Input: part model. Units: mm. Frame: model coordinates. A direction names the side the tool comes from. Coordinates: 2 decimals unless noted, no trailing zeros. Loops run counter-clockwise (first coordinate to the right, second up) from the corner with the lowest first, then second, coordinate; pieces in that order, holes last. Notation, with made-up numbers: (32.5, 85.25) - (76.5, 85.25) arc R26 cw to (76.5, 120.25) - close; hole circle Ø3 at (-9, 63). An arc over 180 degrees is marked (long way). Use a Markdown table: item, result. Add a question column.
1. Section query C-C on y = 4. Return the cut outline in (x, z) (3 decimals).
2. Section query A-A on x = -50.8. Return the cut outline in (y, z), then the cut area to 3 significant figures.
3. Section query B-B on z = -15.24. Return the cut outline in (x, y), then the cut area to 3 significant figures.
4. Ray query, L1, parallel to Z at x = -35.56, y = 1; L2, parallel to X at y = 8.5, z = -30.5; L3, parallel to X at y = 9.75, z = -4. Return the intervals inside material, ascending. Write a range as [from, to].
5. Contact query for flat-ended pins moving along their axis: P1, Ø2.5, axis at y = 6.5, z = 2.5, coming from the -X side; P2, Ø0.6, axis at x = -3.5, z = -4.5, coming from the +Y side; P3, Ø2.5, axis at y = 6, z = -54.5, coming from the +X side. Output: stop coordinate, or through.
6. Draft query along Y for faces 5 (the face through (-3.5, 6, -3)), 6 (the face through (-34.93, 10.09, 1.08)), 7 (the face through (-51, 10, -42)). Return one class per face: released by +Y, released by -Y, zero draft, split by the parting line, or undercut.
7. Access query for faces 1 (the face through (-8, 8, 2)), 2 (the face through (-44.34, 7, -2)), 3 (the face through (-42.565, 6, 1)), 4 (the face through (-38, 7, -10)). Directions: +Z, -Z, +X, -X, +Y, -Y. A direction counts if a zero-diameter tool reaches every point of the face in a straight line with its end or side. Return the directions, or none.
8. Section query D-D on z = -49.5. Return the cut outline in (x, y).
Autodesk Inventor part; units mm, degrees
ref_plane "YZ Plane" through (0, 0, 0) normal (1, 0, 0) x (0, 1, 0)
ref_plane "XZ Plane" through (0, 0, 0) normal (0, 1, 0) x (-1, 0, 0)
ref_plane "XY Plane" through (0, 0, 0) normal (0, 0, 1) x (1, 0, 0)
sketch "Sketch1" plane through (0, 0, 0) normal (0, 1, 0) x (-1, 0, 0)
  line L0 (0, 0) -> (53.34, 0)
  line L1 (53.34, 0) -> (53.34, -66.04)
  line L2 (0, -66.04) -> (0, 0)
  circle A0 centre (50.8, -15.24) radius 1.6
  circle A1 centre (2.54, -15.24) radius 1.6
  circle A2 centre (35.56, -66.04) radius 1.6
  circle A3 centre (7.62, -66.04) radius 1.6
  line L3 (2.54, -66.04) -> (5.08, -68.58)
  line L4 (5.08, -68.58) -> (38.02, -68.58)
  line L5 (38.02, -68.58) -> (40.56, -66.04)
  line L6 (53.34, -66.04) -> (40.56, -66.04)
  line L7 (2.54, -66.04) -> (0, -66.04)
  dimension "d0" = 66.04
  dimension "d1" = 53.34
  dimension "d2" = 3.2
  dimension "d3" = 2.54
  dimension "d4" = 2.54
  dimension "d5" = 45.72
  dimension "d6" = 17.78
  dimension "d7" = 2.54
  dimension "d8" = 2.54
  dimension "d9" = 2.54
  dimension "d10" = 2.54
  dimension "d11" = 15.24
  dimension "d12" = 15.24
  dimension "d13" = 5
extrude "Extrusion1" add sketch "Sketch1" along normal blind 1.5
sketch "Sketch2" plane through (0, 1.5, 0) normal (0, 1, 0) x (1, 0, 0)
  line L0 (-44.34, 10) -> (-32.34, 10)
  line L1 (-32.34, 10) -> (-32.34, -6.5)
  line L2 (-32.34, -6.5) -> (-44.34, -6.5)
  line L3 (-44.34, -6.5) -> (-44.34, 10)
  line L4 (-53.34, 0) -> (0, 0)
  line L5 (-53.34, 66.04) -> (-53.34, 0)
  dimension "d16" = 12
  dimension "d17" = 16.5
  dimension "d18" = 6.5
  dimension "d41" = 9
extrude "Extrusion2" add sketch "Sketch2" along normal blind 11
sketch "Sketch3" plane through (-44.34, 1.5, 6.5) normal (0, 0, 1) x (1, 0, 0)
  line L0 (3.25, 7.025) -> (8.75, 7.025)
  line L1 (8.75, 7.025) -> (8.75, 3.975)
  line L2 (8.75, 3.975) -> (3.25, 3.975)
  line L3 (3.25, 3.975) -> (3.25, 7.025)
  line L4 (1.775, 1.61) -> (10.225, 1.61)
  line L5 (10.225, 1.61) -> (10.225, 7.775)
  line L6 (8.61, 9.39) -> (3.39, 9.39)
  line L7 (1.775, 7.775) -> (1.775, 1.61)
  line L8 (1.775, 7.775) -> (3.39, 9.39)
  line L9 (8.61, 9.39) -> (10.225, 7.775)
  line L10 (12, 0) -> (12, 11)
  line L11 (0, 11) -> (12, 11)
  point P0 (44.34, -1.5)
  dimension "d21" = 8.45
  dimension "d22" = 1.775
  dimension "d23" = 5.5
  dimension "d25" = 1.475
  dimension "d26" = 3.05
  dimension "d27" = 7.78
  dimension "d28" = 45
  dimension "d29" = 45
  dimension "d30" = 2.365
  dimension "d31" = 1.61
  dimension "d32" = 0.75
extrude "Extrusion3" cut sketch "Sketch3" against normal blind 11
sketch "Sketch4" plane through (0, 1.5, 0) normal (0, 1, 0) x (1, 0, 0)
  line L0 (-12.5, 12.3) -> (-3.5, 12.3)
  line L1 (-3.5, 12.3) -> (-3.5, -2)
  line L2 (-3.5, -2) -> (-12.5, -2)
  line L3 (-12.5, -2) -> (-12.5, 12.3)
  line L4 (-32.34, 0) -> (0, 0)
  line L5 (0, 0) -> (0, 66.04)
  dimension "d35" = 9
  dimension "d36" = 14.3
  dimension "d37" = 2
  dimension "d40" = 3.5
extrude "Extrusion4" add sketch "Sketch4" along normal blind 11
sketch "Sketch5" plane through (-12.5, 1.5, 2) normal (0, 0, 1) x (1, 0, 0)
  circle A0 centre (4.5957, 6.5) radius 3.15
  line L0 (0, 0) -> (9, 0)
  circle A1 centre (4.5957, 6.5) radius 1.25
  point P0 (12.5, -1.5)
  dimension "d42" = 6.5
  dimension "d43" = 6.3
  dimension "d44" = 2.5
extrude "Extrusion5" cut sketch "Sketch5" against normal blind 11
sketch "Sketch6" plane through (-3.5, 1.5, -12.3) normal (0, 0, -1) x (-1, 0, 0)
  line L0 (-2.56, 0) -> (0.64, 0)
  line L1 (0.5, 0) -> (0.5, 6)
  line L2 (1.58, 0) -> (34.52, 0)
  line L3 (8.5, 0) -> (8.5, 6)
  arc A0 (8.5, 6) -> (0.5, 6) centre (4.5, 6) ccw
  line L4 (9, 0) -> (9, 11)
  line L5 (0, 11) -> (9, 11)
  line L6 (0, 0) -> (0, 11)
  line L7 (9, 0) -> (0, 0)
  line L8 (9, 0) -> (9, 11)
  line L9 (0, 11) -> (9, 11)
  line L10 (0, 0) -> (0, 11)
  point P0 (-3.5, -1.5)
  dimension "d47" = 8
  dimension "d48" = 8
  dimension "d49" = 0.5
  dimension "d50" = 1
  dimension "d51" = 4.5
extrude "Extrusion6" cut sketch "Sketch6" against normal blind 1 contours L6 L5 L4 L2 L3 A0 L1 L0
sketch "Sketch7" plane through (-3.5, 1.5, -11.3) normal (0, 0, -1) x (-1, 0, 0)
  arc A0 (8.5, 6) -> (0.5, 6) centre (4.5, 6) ccw
  arc A1 (8.5, 6) -> (0.5, 6) centre (4.5, 6) ccw
  line L0 (0.5, 6) -> (0, 6)
  line L1 (0, 0) -> (0, 11)
  line L2 (0, 6) -> (0, 11)
  line L3 (0, 11) -> (9, 11)
  line L4 (9, 11) -> (0, 11)
  line L5 (9, 11) -> (9, 6)
  line L6 (8.5, 0) -> (8.5, 6)
  line L7 (9, 6) -> (8.5, 6)
  point P0 (-3.5, -1.5)
extrude "Extrusion7" cut sketch "Sketch7" against normal blind 9.8
sketch "Sketch8" plane through (0, 1.5, 0) normal (0, 1, 0) x (1, 0, 0)
  line L0 (-3.79, 26.54) -> (-1.29, 26.54)
  line L1 (-1.29, 26.54) -> (-1.29, 65.54)
  line L2 (-1.29, 65.54) -> (-3.79, 65.54)
  line L3 (-3.79, 65.54) -> (-3.79, 26.54)
  line L4 (-52.05, 17.54) -> (-49.55, 17.54)
  line L5 (-49.55, 17.54) -> (-49.55, 65.54)
  line L6 (-49.55, 65.54) -> (-52.05, 65.54)
  line L7 (-52.05, 65.54) -> (-52.05, 17.54)
  circle A0 centre (-50.8, 15.24) radius 1.6
  circle A1 centre (-2.54, 15.24) radius 1.6
  line L8 (0, 66.04) -> (-2.54, 66.04)
  line L9 (-40.56, 66.04) -> (-53.34, 66.04)
  point P0 (0, 0)
  dimension "d56" = 2.5
  dimension "d57" = 2.5
  dimension "d58" = 39
  dimension "d59" = 48
  dimension "d60" = 1.25
  dimension "d61" = 1.25
  dimension "d62" = 0.5
  dimension "d63" = 0.5
extrude "Extrusion8" add sketch "Sketch8" along normal blind 8.5 contours L3 L2 L1 L0 | L7 L6 L5 L4
properties part number "RoughArduino"
Resolved:
| question | item | result |
|---|---|---|
| 1 | outline | (-52.05, -65.54) - (-49.55, -65.54) - (-49.55, -17.54) - (-52.05, -17.54) - close; (-44.34, -10) - (-32.34, -10) - (-32.34, 6.5) - (-34.115, 6.5) - (-34.115, -4.5) - (-42.565, -4.5) - (-42.565, 6.5) - (-44.34, 6.5) - close; (-12.5, -11.3) - (-12, -11.3) - (-12, -12.3) - (-4, -12.3) - (-4, -11.3) - (-3.5, -11.3) - (-3.5, 2) - (-12.5, 2) - close; (-3.79, -65.54) - (-1.29, -65.54) - (-1.29, -26.54) - (-3.79, -26.54) - close |
| 2 | outline | (0, -66.04) - (1.5, -66.04) - (1.5, -65.54) - (10, -65.54) - (10, -17.54) - (1.5, -17.54) - (1.5, -16.84) - (0, -16.84) - close; (0, -13.64) - (1.5, -13.64) - (1.5, 0) - (0, 0) - close |
| 2 | area | 502 mm² |
| 3 | outline | (-53.34, 0) - (-52.4, 0) - (-52.4, 1.5) - (-53.34, 1.5) - close; (-49.2, 0) - (-4.14, 0) - (-4.14, 1.5) - (-49.2, 1.5) - close; (-0.94, 0) - (0, 0) - (0, 1.5) - (-0.94, 1.5) - close |
| 3 | area | 70.4 mm² |
| 4 | L1 | [-68.58, -67.64], [-64.44, 0] |
| 4 | L2 | [-52.05, -49.55], [-3.79, -1.29] |
| 4 | L3 | [-44.34, -42.09], [-34.59, -32.34], [-11.31, -10.52], [-5.29, -4.69] |
| 5 | P1 | x = -44.34 |
| 5 | P2 | y = 7.5 |
| 5 | P3 | x = -1.29 |
| 6 | face 5 | zero draft |
| 6 | face 6 | undercut |
| 6 | face 7 | released by +Y |
| 7 | face 1 | +Z, +X, +Y, -Y |
| 7 | face 2 | +Z, -Z, -X, +Y |
| 7 | face 3 | +Z |
| 7 | face 4 | -Z, -X, +Y |
| 8 | outline | (-53.34, 0) - (0, 0) - (0, 1.5) - (-1.29, 1.5) - (-1.29, 10) - (-3.79, 10) - (-3.79, 1.5) - (-49.55, 1.5) - (-49.55, 10) - (-52.05, 10) - (-52.05, 1.5) - (-53.34, 1.5) - close |
